Autodesk Inventor part; units mm, degrees
ref_plane "YZ Plane" through (0, 0, 0) normal (1, 0, 0) x (0, 1, 0)
ref_plane "XZ Plane" through (0, 0, 0) normal (0, 1, 0) x (-1, 0, 0)
ref_plane "XY Plane" through (0, 0, 0) normal (0, 0, 1) x (1, 0, 0)
sketch "Sketch1" plane through (0, 0, 0) normal (0, 0, 1) x (1, 0, 0)
  circle A0 centre (0, 0) radius 1
  dimension "d0" = 2
extrude "Extrusion1" add sketch "Sketch1" along normal blind 6
thread "Thread1"
sketch "Sketch2" plane through (0, 0, 6) normal (0, 0, 1) x (1, 0, 0)
  circle A0 centre (0, 0) radius 1
  circle A1 centre (0, 0) radius 1.85
  dimension "d6" = 3.7
extrude "Extrusion2" add sketch "Sketch2" along normal blind 1.7 contours A0 | A1
fillet "Fillet1" radius 0.8 1 edges at (-1.85, 0, 7.7)
sketch "Sketch3" plane through (0, 0, 7.7) normal (0, 0, 1) x (1, 0, 0)
  circle A0 centre (0, 0) radius 1.05
  line L0 (-0.35, 1.25) -> (0.35, 1.25)
  line L1 (0.35, 1.25) -> (0.35, -1.25)
  line L2 (0.35, -1.25) -> (-0.35, -1.25)
  line L3 (-0.35, -1.25) -> (-0.35, 1.25)
  line L4 (-1.25, 0.35) -> (1.25, 0.35)
  line L5 (1.25, 0.35) -> (1.25, -0.35)
  line L6 (1.25, -0.35) -> (-1.25, -0.35)
  line L7 (-1.25, -0.35) -> (-1.25, 0.35)
  point P0 (0, 1.25)
  point P1 (0.35, 0)
  point P2 (-1.25, 0)
  point P3 (0, 0.35)
  dimension "d11" = 0.7
  dimension "d15" = 2.5
  dimension "d16" = 0.7
  dimension "d17" = 2.5
extrude "Extrusion3" cut sketch "Sketch3" against normal blind 1 contours A0 L6 L1 L4 | A0 L4 L5 L6 | L1 L4 L3 A0 | A0 L3 L0 L1 | L1 L6 L3 L4 | L1 L2 L3 A0 | A0 L3 L6 L1 | L3 L6 A0 L4 | A0 L6 L7 L4
equation "\"d16\" = d11"
equation "\"d17\" = d15"
properties part number "M2x6 Screw"
Source: CAD feature listing. Evaluate the final solid. Frame: model axes, mm. A direction names the side the tool comes from. Round coordinates to 2 decimals unless told otherwise and drop trailing zeros. Loops run counter-clockwise (first coordinate to the right, second up) from the corner with the lowest first, then second, coordinate; pieces in that order, holes last.
1. Ray query, L1, parallel to Y at x = -0.3, z = 6.75; L2, parallel to Z at x = 0.75, y = -0.05; L3, parallel to X at y = -0.15, z = 5.75. Return the intervals inside material, ascending.
2. Section query D-D on z = 6.5. Output: boundary loops of the cut face in (x, y).
3. Section query A-A on y = 0. Output: boundary loops of the cut face in (x, z), and give its area (3 significant figures).
4. Section query C-C on z = 2.25. Output: boundary loops of the cut face in (x, y), and give its area (3 significant figures).
5. Access query for faces 1 (the flat face through (0, 0, 0)), 2 (the flat face through (1, -0.35, 7)), 3 (the cylindrical face through (0, 1, 3)). Directions: +Z, -Z, +X, -X, +Y, -Y. A direction counts if a zero-diameter tool reaches every point of the face in a straight line with its end or side. Return the directions, or none.
6. Mould query, pull axis Y, two halves, no side actions, for faces 4 (the cylindrical face through (-0.401, 1.806, 6.444)), 5 (the flat face through (-0.35, 1, 7)), 6 (the flat face through (1, -1, 6)). Classes: released by +Y, released by -Y, zero draft, split by the parting line, or undercut.
7. Contact query for flat-ended pins moving along their axis: pin 1 (0.5 mm diameter, centred on x = 1, z = 7.5, fed in from +Y); pin 2 (0.6 mm diameter, centred on x = 0, z = 7.5, fed in from +Y); pin 3 (0.7 mm diameter, centred on y = -0.5, z = 7, fed in from +X). Output: stop coordinate, or through.
Answers below:
1. L1: y = -1.83 to -1.25, 1.25 to 1.83
1. L2: z = 0 to 6.7
1. L3: x = -0.99 to 0.99
2. outline: circle Ø3.7 at (0, 0)
3. outline: (-1.85, 6) - (-1, 6) - (-1, 0) - (1, 0) - (1, 6) - (1.85, 6) - (1.85, 6.9) arc R0.8 ccw to (1.25, 7.67) - (1.25, 6.7) - (-1.25, 6.7) - (-1.25, 7.67) arc R0.8 ccw to (-1.85, 6.9) - close
3. area: 15.5 mm2
4. outline: circle Ø2 at (0, 0)
4. area: 3.14 mm2
5. face 1: -Z, +X, -X, +Y, -Y
5. face 2: +Z
5. face 3: -Z
6. face 4: split by the parting line
6. face 5: undercut
6. face 6: zero draft
7. pin 1: stops at y = 1.52
7. pin 2: stops at y = 1.79
7. pin 3: stops at x = 1.84
